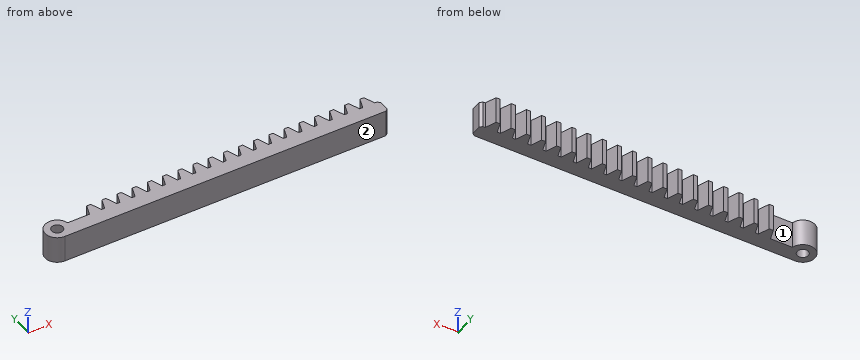
```python
from build123d import *

# Parameters (mm, degrees)
SKETCH_1_W             = 60
SKETCH_1_H             = 3
EXTRUDE_1_DEPTH        = 5.5
EXTRUDE_2_DEPTH        = 5.5
PATTERN_LINEAR_1_COUNT = 19
PATTERN_LINEAR_1_PITCH = 3.141592654
SKETCH_3_R             = 1.15
EXTRUDE_1_2_DEPTH      = 5.5
CUT_EXTRUDE_2_DEPTH    = 6


with BuildPart() as part:
    # 草图1 → Extrude 1 (new body)
    with BuildSketch(Plane.XY):
        with Locations((30, -1.5)):
            Rectangle(SKETCH_1_W, SKETCH_1_H)
    extrude(amount=EXTRUDE_1_DEPTH)

    # 草图2 → 拉伸2 (add)
    with BuildSketch(Plane.XY.offset(5.5)):
        Polygon((0, 0), (0.818933027, 2.25), (1.661788885, 2.25), (2.480721912, 0), align=None)
    extrude_2 = extrude(amount=-EXTRUDE_2_DEPTH)

    # 阵列(线性)1: 拉伸2 ×19
    with Locations(*[(i * PATTERN_LINEAR_1_PITCH, 0, 0) for i in range(1, PATTERN_LINEAR_1_COUNT)]):
        add(extrude_2)

    # 草图3 → Extrude 1 2 (add)
    with BuildSketch(Plane(origin=(0, 0, 0), x_dir=(-1, 0, 0), z_dir=(0, 0, -1))):
        with BuildLine():
            Line((7, -3), (0, -3))
            Line((0, -3), (0, 0))
            Line((0, 0), (4.550510054, 0))
            ThreePointArc((4.550510054, 0), (8.93649166, 1.081138846), (7, -3))
        make_face()
        with Locations((7, -0.5)):
            Circle(SKETCH_3_R, mode=Mode.SUBTRACT)
    extrude(amount=-EXTRUDE_1_2_DEPTH)

    # 草图5 → 切除-拉伸2 (cut)
    with BuildSketch(Plane(origin=(0, 0, 0), x_dir=(-1, 0, 0), z_dir=(0, 0, -1))):
        Polygon((-59.514694839, 0), (-60, -0.5), (-60, 0), align=None)
        Polygon((-60, -3), (-60, -2.5), (-59.5, -3), align=None)
    extrude(amount=-CUT_EXTRUDE_2_DEPTH, mode=Mode.SUBTRACT)


solid = part.part
```
Geometry: final body of the model. Coordinates: model frame, mm. Face numbers are marked on the shaded views. Round coordinates to 2 decimals unless told otherwise and drop trailing zeros. Write each question's results on one line, items separated by ' | '.
Item 1: Line query: probe 1 along Y at (x, z) = (-7, 3.4); probe 2 along Y at (x, z) = (12, 4.4); probe 3 along X at (y, z) = (-1.15, 2.55). Output: solid intervals per line, ascending. Write a range as [from, to].
Answers below:
probe 1: y = [-3, -1.65], [0.65, 2] | probe 2: y = [-3, 0] | probe 3: x = [-9.41, -7.95], [-6.05, 60]
Item 2: Pin query (flat end, axial travel): pin 1 Ø2 at (x, y) = (16.5, -1.5) entering from -Z; pin 2 Ø0.5 at (x, z) = (18.5, 3.5) entering from +Y. Return the tip coordinate at first contact, or that it passes through.
Answers below:
pin 1: stops at z = 0 | pin 2: stops at y = 0
Item 3: Pull-direction query (X, two-part tool) for the marked faces 1 and 2; classes: pulls with the +X half, pulls with the -X half, needs draft (parallel to the pull), parting line crosses it, or undercut.
Answers below:
face 1: undercut | face 2: needs draft
